Part model, mm, in its own coordinate system. A direction names the side the tool comes from. Coordinates: 2 decimals unless noted, no trailing zeros. Order: outer loops, then holes, each group sorted by start corner. A loop starts at its lowest first (then second) coordinate and runs counter-clockwise, first axis right, second up.
```python
from build123d import *

# Parameters (mm, degrees)
SKETCH1_W           = 33
SKETCH1_H           = 33
BOSS_EXTRUDE1_DEPTH = 20
SKETCH2_R           = 16
CUT_EXTRUDE1_DEPTH  = 3
SKETCH3_R           = 1
CUT_EXTRUDE2_DEPTH  = 2
FILLET1_R           = 1


with BuildPart() as part:
    # Sketch1 → Boss-Extrude1 (new body)
    with BuildSketch(Plane(origin=(0, 0, 0), x_dir=(1, 0, 0), z_dir=(0, 1, 0))):
        Rectangle(SKETCH1_W, SKETCH1_H)
    extrude(amount=BOSS_EXTRUDE1_DEPTH)

    # Sketch2 → Cut-Extrude1 (cut)
    with BuildSketch(Plane(origin=(0, 20, 0), x_dir=(1, 0, 0), z_dir=(0, 1, 0))):
        Circle(SKETCH2_R)
    extrude(amount=-CUT_EXTRUDE1_DEPTH, mode=Mode.SUBTRACT)

    # Sketch3 → Cut-Extrude2 (cut)
    with BuildSketch(Plane.XZ):
        Circle(SKETCH3_R)
    extrude(amount=-CUT_EXTRUDE2_DEPTH, mode=Mode.SUBTRACT)

    # Fillet1
    fillet1_edges = [part.edges().sort_by_distance(p)[0] for p in [
        (-1, 2, 0),
    ]]
    fillet(fillet1_edges, radius=FILLET1_R)


solid = part.part
```
(1) Probe line 1 (X direction, y = 19.15, z = 0); line 2 (Z direction, x = 0, y = 0.4). List the from-to ranges inside material, lowest first.
(2) Pull direction X, two halves, no side cores. Call faces 3 (the face through (16.5, 10, 0)), 4 (the face through (-0.217, 0.493, -0.976)), 5 (the face through (0, 0, -4)), 6 (the face through (-3.47, 18.52, 15.62)): +X half, -X half, draft (parallel to the pull), parting line (faces both ways), or undercut.
(3) Slice it at A-A, the plane y = 18.5. Give the cut face in (x, z), then the cut area to 3 significant figures.
(4) Slice it at B-B, the plane x = 0. Give the cut face in (y, z), then the cut area to 3 significant figures.
(5) Slice it at D-D, the plane z = 4. Give the cut face in (x, y), then the cut area to 3 significant figures.
(6) Tool access for faces 1 (the face through (0, 17, 0)), 2 (the face through (-16.5, 10, 0)): list every direction of +Z, -Z, +X, -X, +Y, -Y with a clear straight run to the whole face (end or side of a thin tool).
(7) Drop a flat-ended pin along its axis: pin 1 (9.5 mm diameter, centred on x = 4.5, z = 2.5, fed in from +Y). Give the stop position or say it passes through.
(8) Slice it at C-C, the plane z = 0. Give the cut face in (x, y), then the cut area to 3 significant figures.
Here are the results:
1. line 1: x = -16.5 to -16, 16 to 16.5
1. line 2: z = -16.5 to -1, 1 to 16.5
2. face 3: +X half
2. face 4: undercut
2. face 5: draft
2. face 6: undercut
3. outline: (-16.5, -16.5) - (16.5, -16.5) - (16.5, 16.5) - (-16.5, 16.5) - close; hole circle Ø32 at (0, 0)
3. area: 285 mm2
4. outline: (0, -16.5) - (20, -16.5) - (20, -16) - (17, -16) - (17, 16) - (20, 16) - (20, 16.5) - (0, 16.5) - (0, 1) - (1, 1) arc R1 cw to (1, -1) - (0, -1) - close
4. area: 560 mm2
5. outline: (-16.5, 0) - (16.5, 0) - (16.5, 20) - (15.49, 20) - (15.49, 17) - (-15.49, 17) - (-15.49, 20) - (-16.5, 20) - close
5. area: 567 mm2
6. face 1: +Y
6. face 2: +Z, -Z, -X, +Y, -Y
7. pin 1: stops at y = 17
8. outline: (-16.5, 0) - (-1, 0) - (-1, 1) arc R1 cw to (1, 1) - (1, 0) - (16.5, 0) - (16.5, 20) - (16, 20) - (16, 17) - (-16, 17) - (-16, 20) - (-16.5, 20) - close
8. area: 560 mm2
